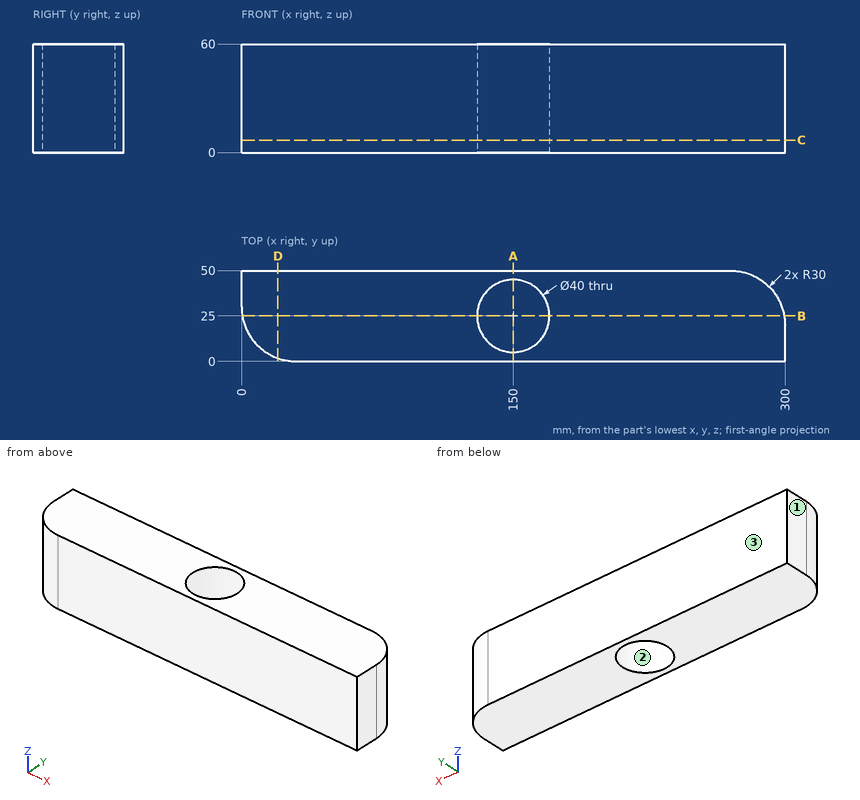
Here's the drawing with two shaded views (mm, measured from the low corner). I have some questions. Round coordinates to 2 decimals unless told otherwise and drop trailing zeros. Loops run counter-clockwise (first coordinate to the right, second up) from the corner with the lowest first, then second, coordinate; pieces in that order, holes last.
1. If I drill on probe 1 along Y at (x, z) = (150, 47.5); probe 2 along X at (y, z) = (23, 39); probe 3 along Y at (x, z) = (134.5, 47), over which ranges is the centre line in solid material (lowest first)?
Answers:
probe 1: y = 0 to 5, 45 to 50
probe 2: x = 0.83 to 130.1, 169.9 to 299.85
probe 3: y = 0 to 12.36, 37.64 to 50
2. Suppose I cut it at D-D, the plane x = 20. Please give me the cut outline in (y, z), and give its area (3 significant figures).
Answers:
outline: (1.72, 0) - (50, 0) - (50, 60) - (1.72, 60) - close
area: 2,900 mm2
3. Suppose I cut it at B-B, the plane y = 25. Please give me the cut outline in (x, z), and give its area (3 significant figures).
Answers:
outline: (0.42, 0) - (130, 0) - (130, 60) - (0.42, 60) - close; (170, 0) - (299.58, 0) - (299.58, 60) - (170, 60) - close
area: 15,500 mm2
4. Will these pins go through, and if not, where does the flat tip stop? pin 1 (2 mm diameter, centred on y = 39, z = 27, fed in from +X); pin 2 (6 mm diameter, centred on y = 37, z = 46, fed in from +X).
Answers:
pin 1: stops at x = 294
pin 2: stops at x = 296.53
5. Thinking about a two-plate mould opening in X: for the marked faces 1, 2 and 3, which applies, released by +X, released by -X, zero draft, split by the parting line, or undercut?
Answers:
face 1: released by -X
face 2: undercut
face 3: zero draft
6. Suppose I cut it at A-A, the plane x = 150. Please give me the cut outline in (y, z), and give its area (3 significant figures).
Answers:
outline: (0, 0) - (5, 0) - (5, 60) - (0, 60) - close; (45, 0) - (50, 0) - (50, 60) - (45, 60) - close
area: 600 mm2
7. Suppose I cut it at C-C, the plane z = 7. Please give me the cut outline in (x, y).
Answers:
outline: (0, 30) arc R30 ccw to (30, 0) - (300, 0) - (300, 20) arc R30 ccw to (270, 50) - (0, 50) - close; hole circle Ø40 at (150, 25)
